Could you check a few things on this drawing? It's one solid part, dimensions in mm from its lowest x, y, z. Give positions to 0.01 mm unless a question says otherwise; leave off trailing zeros. Loops run counter-clockwise (first coordinate to the right, second up) from the corner with the lowest first, then second, coordinate; pieces in that order, holes last. Notation, with made-up numbers: (83, -10) - (133, -10) arc R34 cw to (133, 25) - close; hole circle Ø7 at (73, -32.5). An arc over 180 degrees is marked (long way). Write each question's results on one line, items separated by ' | '. Start each with the question number.
(1) I need wall thicknesses on line 1 (X direction, y = 38, z = 0.3); line 2 (Y direction, x = 19.75, z = 0.8); line 3 (Z direction, x = 4.5, y = 34). Which ranges of each line are inside material? Lowest first, please.
(2) For pin 1 (3 mm diameter, centred on x = 3.5, y = 38, fed in from -Z); pin 2 (10 mm diameter, centred on x = 7, y = 21.5, fed in from +Z); pin 3 (1.5 mm diameter, centred on y = 8.5, z = 3, fed in from +X), each with a flat end and sliding along its axis, tell me the tip position at first contact or that it passes through.
(3) Suppose I cut it at D-D (y = 12). Please give me the cut outline in (x, z).
(4) Suppose I cut it at A-A (z = 0.55). Please give me the cut outline in (x, y).
(5) Suppose I cut it at B-B (y = 3). Please give me the cut outline in (x, z), and give its area (3 significant figures).
(6) Suppose I cut it at C-C (x = 11.5). Please give me the cut outline in (y, z), and give its area (3 significant figures).
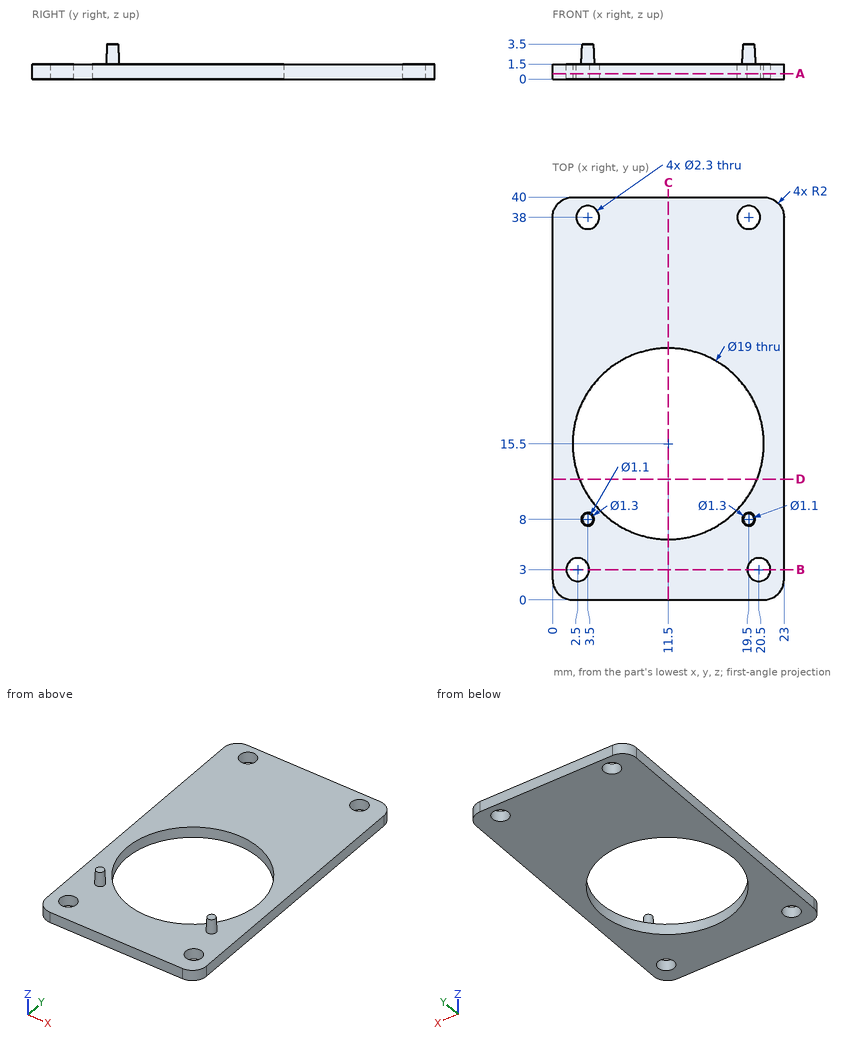
Output values:
1) line 1: 0 to 2.35, 4.65 to 18.35, 20.65 to 23 | line 2: 0 to 2.13, 3.87 to 10.79, 20.21 to 36.88, 39.12 to 40 | line 3: 0 to 1.5
2) pin 1: z = 0 | pin 2: z = 1.5 | pin 3: x = 20.1
3) outline: (0, 0) - (2.67, 0) - (2.67, 1.5) - (0, 1.5) - close; (20.33, 0) - (23, 0) - (23, 1.5) - (20.33, 1.5) - close
4) outline: (0, 2) arc R2 ccw to (2, 0) - (21, 0) arc R2 ccw to (23, 2) - (23, 38) arc R2 ccw to (21, 40) - (2, 40) arc R2 ccw to (0, 38) - close; hole circle Ø2.3 at (2.5, 3); hole circle Ø19 at (11.5, 15.5); hole circle Ø2.3 at (3.5, 38); hole circle Ø2.3 at (19.5, 38); hole circle Ø2.3 at (20.5, 3)
5) outline: (0, 0) - (1.35, 0) - (1.35, 1.5) - (0, 1.5) - close; (3.65, 0) - (19.35, 0) - (19.35, 1.5) - (3.65, 1.5) - close; (21.65, 0) - (23, 0) - (23, 1.5) - (21.65, 1.5) - close | area: 27.6 mm2
6) outline: (0, 0) - (6, 0) - (6, 1.5) - (0, 1.5) - close; (25, 0) - (40, 0) - (40, 1.5) - (25, 1.5) - close | area: 31.5 mm2
